Can you work these out from the model? Positions are in its coordinate system, mm. Face numbers are marked on the shaded views. A direction names the side the tool comes from. Give positions to 0.01 mm unless a question says otherwise; leave off trailing zeros. Loops run counter-clockwise (first coordinate to the right, second up) from the corner with the lowest first, then second, coordinate; pieces in that order, holes last. Notation, with made-up numbers: (10, 75) -> (54, 75) arc R24 ccw to (54, 112) -> close; hole circle Ø4 at (57, 16). An arc over 180 degrees is marked (long way). Use CSV: the item, a comma, the result in double quotes.
from build123d import *

# Parameters (mm, degrees)
SKETCH1_W           = 48
SKETCH1_H           = 36
SKETCH1_R           = 1.7
BOSS_EXTRUDE1_DEPTH = 14
SKETCH2_R           = 1.5
SKETCH2_R_2         = 3.1
CUT_EXTRUDE3_DEPTH  = 15
SKETCH5_R           = 15
CUT_EXTRUDE4_DEPTH  = 3
SKETCH7_R           = 4.75
CUT_EXTRUDE5_DEPTH  = 6
FILLET1_R           = 16
FILLET2_R           = 16
FILLET3_R           = 0.5
CHAMFER2_SIZE       = 1


with BuildPart() as part:
    # Sketch1 → Boss-Extrude1 (new body)
    with BuildSketch(Plane(origin=(0, 0, 0), x_dir=(1, 0, 0), z_dir=(0, 1, 0))):
        Rectangle(SKETCH1_W, SKETCH1_H)
        with Locations((-12, 9.75)):
            Circle(SKETCH1_R, mode=Mode.SUBTRACT)
        with Locations((-12, -9.75)):
            Circle(SKETCH1_R, mode=Mode.SUBTRACT)
        with Locations((12, 0)):
            Circle(SKETCH1_R, mode=Mode.SUBTRACT)
    extrude(amount=BOSS_EXTRUDE1_DEPTH)

    # Sketch2 → Cut-Extrude3 (cut, through all)
    with BuildSketch(Plane.XZ):
        with Locations((0, 8)):
            Circle(SKETCH2_R)
        with Locations((0, -8)):
            Circle(SKETCH2_R)
        Circle(SKETCH2_R_2)
    extrude(amount=-CUT_EXTRUDE3_DEPTH, mode=Mode.SUBTRACT)

    # Sketch5 → Cut-Extrude4 (cut)
    with BuildSketch(Plane.XZ):
        Circle(SKETCH5_R)
    extrude(amount=-CUT_EXTRUDE4_DEPTH, mode=Mode.SUBTRACT)

    # Sketch7 → Cut-Extrude5 (cut)
    with BuildSketch(Plane.XZ):
        with Locations((12, 0)):
            Circle(SKETCH7_R)
        with Locations((-12, 9.75)):
            Circle(SKETCH7_R)
        with Locations((-12, -9.75)):
            Circle(SKETCH7_R)
    extrude(amount=-CUT_EXTRUDE5_DEPTH, mode=Mode.SUBTRACT)

    # Fillet1
    fillet1_edges = [part.edges().sort_by_distance(p)[0] for p in [
        (24, 7, 18),
        (24, 7, -18),
    ]]
    fillet(fillet1_edges, radius=FILLET1_R)

    # Fillet2
    fillet2_edges = [part.edges().sort_by_distance(p)[0] for p in [
        (-24, 7, 18),
        (-24, 7, -18),
    ]]
    fillet(fillet2_edges, radius=FILLET2_R)

    # Fillet3
    fillet3_edges = [part.edges().sort_by_distance(p)[0] for p in [
        (5.27456542, 0, -14.042042573),
        (5.27456542, 0, 14.042042573),
        (-15, 0, 0),
        (16.13087492, 0, 2.344860848),
        (-15.686541501, 0, 12.745314969),
        (-15.686541501, 0, -12.745314969),
    ]]
    fillet(fillet3_edges, radius=FILLET3_R)

    # Chamfer2
    chamfer2_edges = [part.edges().sort_by_distance(p)[0] for p in [
        (0, 14, -18),
        (19.313708499, 14, -13.313708499),
        (19.313708499, 14, 13.313708499),
        (0, 14, 18),
        (-24, 14, 0),
        (-19.313708499, 14, -13.313708499),
        (-19.313708499, 14, 13.313708499),
        (24, 14, 0),
    ]]
    chamfer(chamfer2_edges, length=CHAMFER2_SIZE)


solid = part.part
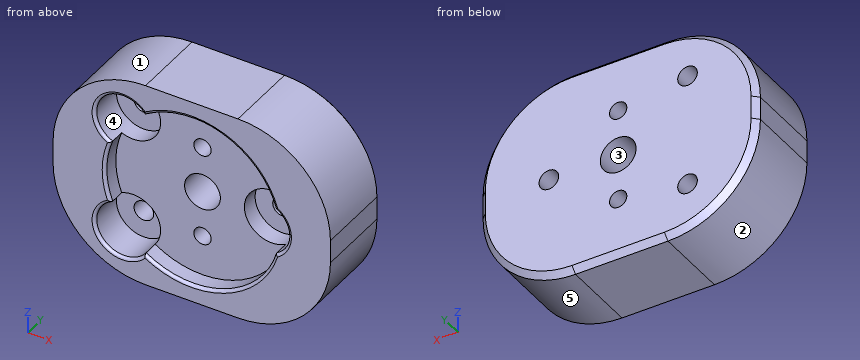
(1) We'd pull the mould along Z, two halves only. Please class the marked faces 1, 2 and 3: released by +Z, released by -Z, zero draft, split by the parting line, or undercut.
Answer sheet:
face 1,"released by +Z"
face 2,"released by -Z"
face 3,"undercut"
(2) Will these pins go through, and if not, where does the flat tip stop? pin 1 Ø3 at (x, z) = (-12, 9.75) entering from +Y; pin 2 Ø5 at (x, z) = (13, 0) entering from -Y; pin 3 Ø4 at (x, y) = (-14.5, 5.5) entering from -Z; pin 4 Ø1 at (y, z) = (4, 8) entering from -X (3 decimals).
Answer sheet:
pin 1,"passes through"
pin 2,"stops at y = 6"
pin 3,"stops at z = -17.35"
pin 4,"stops at x = -23.025"
(3) If we section it at B-B, the plane y = 5.5: Write out the boundary of the cut face in (x, z).
Answer sheet:
outline,"(-24, -2) arc R16 ccw to (-8, -18) -> (8, -18) arc R16 ccw to (24, -2) -> (24, 2) arc R16 ccw to (8, 18) -> (-8, 18) arc R16 ccw to (-24, 2) -> close; hole circle Ø9.5 at (-12, -9.75); hole circle Ø9.5 at (-12, 9.75); hole circle Ø6.2 at (0, 0); hole circle Ø3 at (0, -8); hole circle Ø3 at (0, 8); hole circle Ø9.5 at (12, 0)"
(4) If we section it at C-C, the plane y = 2.5: Write out the boundary of the cut face in (x, z), then the cut area to 3 significant figures.
Answer sheet:
outline,"(-24, -2) arc R16 ccw to (-8, -18) -> (8, -18) arc R16 ccw to (24, -2) -> (24, 2) arc R16 ccw to (8, 18) -> (-8, 18) arc R16 ccw to (-24, 2) -> close; hole (-13.98, -5.43) arc R4.75 ccw (long way) to (-8.18, -12.57) arc R15 ccw to (14.43, -4.08) arc R4.75 ccw to (14.43, 4.08) arc R15 ccw to (-8.18, 12.57) arc R4.75 ccw (long way) to (-13.98, 5.43) arc R15 ccw to start"
area,"707 mm2"
(5) If we section it at A-A, the plane z = 0: Write out the boundary of the cut face in (x, y), then the cut area to 3 significant figures.
Answer sheet:
outline,"(-24, 0) -> (-15.5, 0) arc R0.5 ccw to (-15, 0.5) -> (-15, 3) -> (-3.1, 3) -> (-3.1, 14) -> (-23, 14) -> (-24, 13) -> close; (3.1, 3) -> (7.25, 3) -> (7.25, 6) -> (10.3, 6) -> (10.3, 14) -> (3.1, 14) -> close; (13.7, 6) -> (16.75, 6) -> (16.75, 0.5) arc R0.5 ccw to (17.25, 0) -> (24, 0) -> (24, 13) -> (23, 14) -> (13.7, 14) -> close"
area,"452 mm2"
(6) If I drill on L1, parallel to Y at x = -1.5, z = 13.5; L2, parallel to Z at x = 12, y = 12.5; L3, parallel to Z at x = -12, y = 12.25, over which ranges is the centre line in solid material (lowest first)? Write a range as from..to.
Answer sheet:
L1,"y = 3..14"
L2,"z = -17.49..-1.7, 1.7..17.49"
L3,"z = -17.49..-11.45, -8.05..8.05, 11.45..17.49"
(7) If we section it at D-D, the plane x = -12: Give the number of separate pieces and of enclosed holes in the cut face, then the cut area to 3 significant figures.
Answer sheet:
separate pieces,"3"
enclosed holes,"0"
area,"290 mm2"
(8) Which directions (+Z, -Z, +X, -X, +Y, -Y) give clear straight access to the entire face, cutting with the end or side of a thin tool? Please do the marked faces 4 and 5.
Answer sheet:
face 4,"-Y"
face 5,"-Z, +X, +Y, -Y"
